Input: part model. Units: mm. Frame: model coordinates. Face numbers are marked on the shaded views. A direction names the side the tool comes from. Round coordinates to 2 decimals unless told otherwise and drop trailing zeros. Loops run counter-clockwise (first coordinate to the right, second up) from the corner with the lowest first, then second, coordinate; pieces in that order, holes last. Notation, with made-up numbers: M -9.75,74.5 L 7.25,74.5 A33 ccw 7.25,109.5 Z; hole C -24,27.5 d5. An arc over 180 degrees is marked long. Use one line per item in the form item = value. Start each with the question number.
Q1. Section query A-A, the plane x = 9.25. Output: boundary loops of the cut face in (y, z), and give its area (3 significant figures).
Q2. Ray query, line 1 along Y through (x, z) = (-3, 8.75); line 2 along X through (y, z) = (-21, 1.5); line 3 along Z through (x, y) = (2, -1). Return the intervals inside material, ascending.
Q3. First-contact query: P1, Ø12, axis at y = -18.5, z = 9, coming from the -X side; P2, Ø1.5, axis at x = -0.5, z = 10.5, coming from the +Y side; P3, Ø5, axis at x = -6, z = 0, coming from the -Y side; P4, Ø1.5, axis at x = -0.5, y = -2, coming from the +Z side. Flat tips, straight axial feed; report the tip coordinate or a pass-through.
Q4. Section query D-D, the plane x = -7.5. Output: boundary loops of the cut face in (y, z), and give its area (3 significant figures).
Q5. Access query for the marked faces 1 and 2. Directions: +Z, -Z, +X, -X, +Y, -Y. A direction counts if a zero-diameter tool reaches every point of the face in a straight line with its end or side. Return the directions, or none.
Q6. Section query B-B, the plane z = -5.5. Output: boundary loops of the cut face in (x, y).
Q7. Section query C-C, the plane y = -12.5. Output: boundary loops of the cut face in (x, z).
```python
from build123d import *

# Parameters (mm, degrees)
F0_W     = 22
F0_H     = 25
F1_DEPTH = 3
F3_DEPTH = 2.5
F4_SIZE  = 25


with BuildPart() as f1:
    # F0 (on Front) → F1 (new body)
    with BuildSketch(Plane.XZ):
        Rectangle(F0_W, F0_H)
    extrude(amount=F1_DEPTH)

    # F2 (on face) → F3 (join)
    with BuildSketch(Plane.YZ.offset(11)):
        Polygon((-3, -12.5), (-3, 12.5), (-33, 15.12466), (-33, -12.5), align=None)
    extrude(amount=-F3_DEPTH)

    # F4
    f4_edges = [f1.edges().sort_by_distance(p)[0] for p in [
        (9.75, -33, -12.5),
    ]]
    chamfer(f4_edges, length=F4_SIZE)


solid = f1.part
```
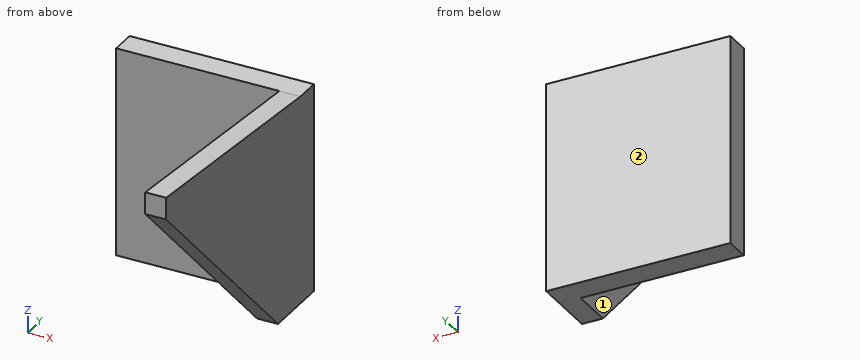
Results found:
q1.outline = M -33,12.5 L -8,-12.5 L 0,-12.5 L 0,12.5 L -3,12.5 L -33,15.12 Z
q1.area = 552 mm²
q2.line_1 = -3 to 0
q2.line_2 = 8.5 to 11
q2.line_3 = -12.5 to 12.5
q3.P1 = 8.5
q3.P2 = 0
q3.P3 = -3
q3.P4 = 12.5
q4.outline = M -3,-12.5 L 0,-12.5 L 0,12.5 L -3,12.5 Z
q4.area = 75.0 mm²
q5.face_1 = +Z, -Z, -X, -Y
q5.face_2 = +Z, -Z, +X, -X, +Y
q6.outline = M -11,-3 L 8.5,-3 L 8.5,-15 L 11,-15 L 11,0 L -11,0 Z
q7.outline = M 8.5,-8 L 11,-8 L 11,13.33 L 8.5,13.33 Z
